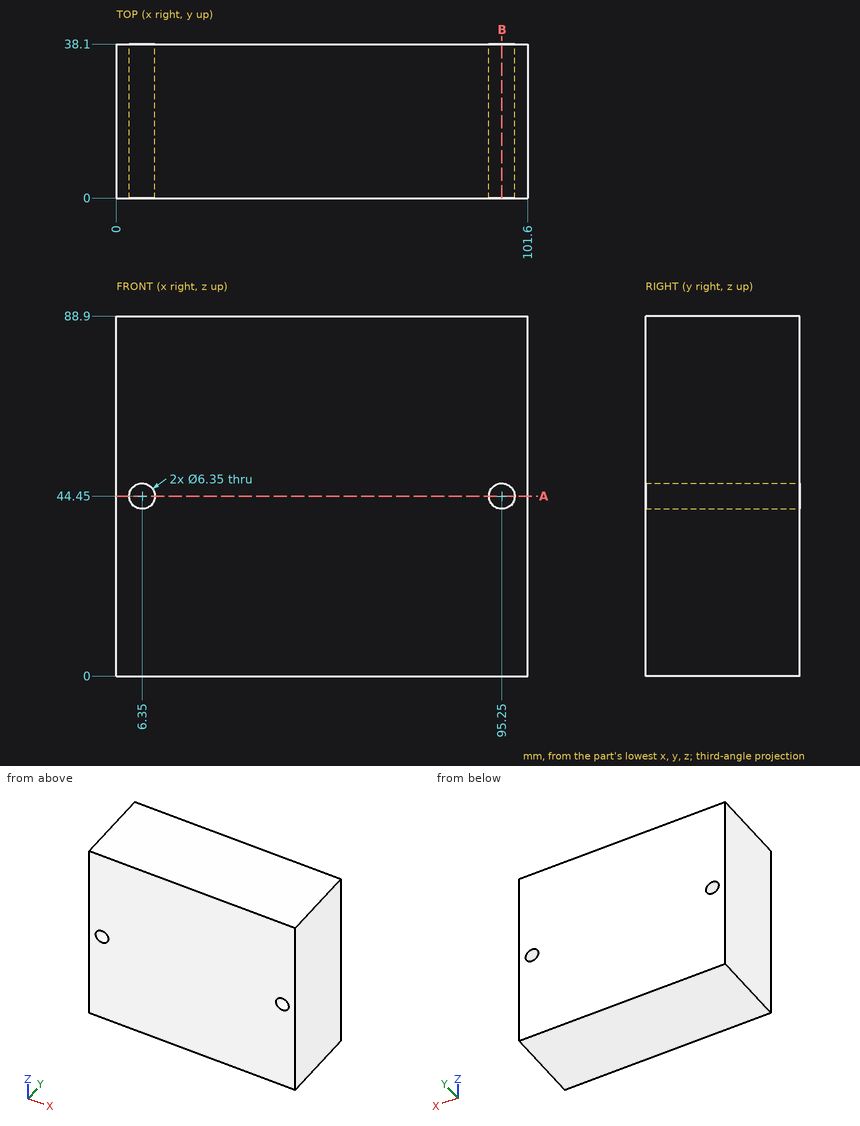
Design review of the part shown in the three views and the two pictorial views. Dimensions are in mm from the part's minimum x, y and z. Coordinates: 2 decimals unless noted, no trailing zeros. Write each loop counter-clockwise with the first axis right and the second up, starting at its lowest first coordinate (ties: lowest second). Pieces come first, ordered by that corner, then holes.
(1) Add section B-B on x = 95.25. Give the boundary of the cut face in (y, z) (3 decimals), then the cut area to 3 significant figures.
(2) Wall thickness on probe 1 along Z at (x, y) = (95, 26); probe 2 along X at (y, z) = (17, 44); probe 3 along X at (y, z) = (36, 43.5): over which ranges is each line inside the solid? List them lowest first.
(3) Add section A-A on z = 44.45. Give the boundary of the cut face in (x, y) (3 decimals).
Answer sheet:
1. outline: (0, 0) - (38.1, 0) - (38.1, 41.275) - (0, 41.275) - close; (0, 47.625) - (38.1, 47.625) - (38.1, 88.9) - (0, 88.9) - close
1. area: 3,150 mm2
2. probe 1: z = 0 to 41.28, 47.62 to 88.9
2. probe 2: x = 0 to 3.21, 9.49 to 92.11, 98.39 to 101.6
2. probe 3: x = 0 to 3.32, 9.38 to 92.22, 98.28 to 101.6
3. outline: (0, 0) - (3.175, 0) - (3.175, 38.1) - (0, 38.1) - close; (9.525, 0) - (92.075, 0) - (92.075, 38.1) - (9.525, 38.1) - close; (98.425, 0) - (101.6, 0) - (101.6, 38.1) - (98.425, 38.1) - close
